The listing builds one solid part. Answer for the finished solid, in the listing's coordinates (mm). Face numbers are marked on the shaded views. Coordinates: 2 decimals unless noted, no trailing zeros. Order: outer loops, then holes, each group sorted by start corner. A loop starts at its lowest first (then second) coordinate and runs counter-clockwise, first axis right, second up. Notation, with made-up numbers: (73, 62.25) - (77, 62.25) arc R31 ccw to (77, 96.25) - close; hole circle Ø10 at (37.5, 76). An arc over 180 degrees is marked (long way). Use a Markdown table: item, result. Add a question column.
Item 1: Find the intervals of material crossed by line 1 along Y through (x, z) = (-76.2, 17.25); line 2 along Y through (x, z) = (68.5, 46); line 3 along X through (y, z) = (3, 30.5), in increasing order.
Item 2: The part is cut by section C-C, the plane y = -7. Give the vertices of the cut face in (x, z), then the cut area to 3 significant figures.
Item 3: Flat-ended cylindrical pins translate along their axes: P1, Ø12.5, axis at x = -75, y = -4, coming from the +Z side; P2, Ø1.9, axis at x = 76.2, y = 0, coming from the -Z side. Find the tip coordinate at first contact, or state that the pin passes through.
Item 4: The part is cut by section B-B, the plane x = -147.5. Give the vertices of the cut face in (y, z), then the cut area to 3 significant figures.
Item 5: The part is cut by section A-A, the plane z = 44.5. Give the vertices of the cut face in (x, y), then the cut area to 3 significant figures.
Item 6: The mould has two halves that part along Y. Classify the marked faces 1, 2, 3 and 4: released by +Y, released by -Y, zero draft, split by the parting line, or undercut.
from build123d import *

# Parameters (mm, degrees)
F0_W     = 381
F0_H     = 76.2
F1_DEPTH = 50.8
F2_W     = 330.2
F2_H     = 25.4
F3_DEPTH = 25.4
F5_D     = 3.175


with BuildPart() as f1:
    # F0 (on Top) → F1 (new body)
    with BuildSketch(Plane.XY):
        Rectangle(F0_W, F0_H)
    extrude(amount=F1_DEPTH)

    # F2 (on face) → F3 (cut)
    with BuildSketch(Plane.XY.offset(50.8)):
        Rectangle(F2_W, F2_H)
    extrude(amount=-F3_DEPTH, mode=Mode.SUBTRACT)

    # F5 (through all)
    with Locations(Plane(origin=(0, 0, 0), x_dir=(1, 0, 0), z_dir=(0, 0, -1))):
        with Locations((-76.2, 0), (76.2, 0)):
            Hole(F5_D / 2)


solid = f1.part
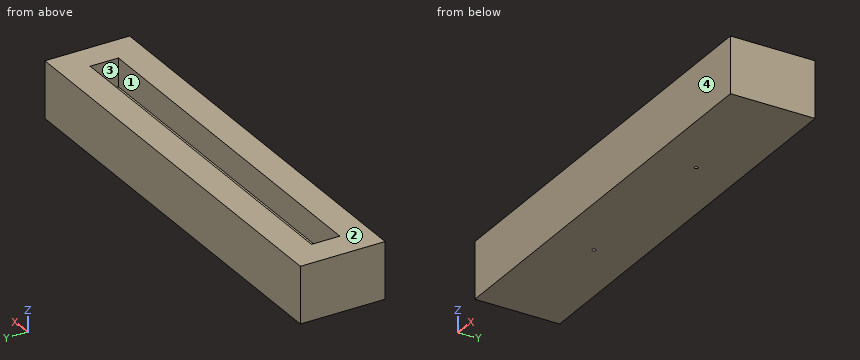
Solution:
| question | item | result |
|---|---|---|
| 1 | line 1 | y = -38.1 to -1.59, 1.59 to 38.1 |
| 1 | line 2 | y = -38.1 to -12.7, 12.7 to 38.1 |
| 1 | line 3 | x = -190.5 to -165.1, 165.1 to 190.5 |
| 2 | outline | (-190.5, 0) - (190.5, 0) - (190.5, 50.8) - (165.1, 50.8) - (165.1, 25.4) - (-165.1, 25.4) - (-165.1, 50.8) - (-190.5, 50.8) - close |
| 2 | area | 11,000 mm2 |
| 3 | P1 | stops at z = 25.4 |
| 3 | P2 | passes through |
| 4 | outline | (-38.1, 0) - (38.1, 0) - (38.1, 50.8) - (12.7, 50.8) - (12.7, 25.4) - (-12.7, 25.4) - (-12.7, 50.8) - (-38.1, 50.8) - close |
| 4 | area | 3,230 mm2 |
| 5 | outline | (-190.5, -38.1) - (190.5, -38.1) - (190.5, 38.1) - (-190.5, 38.1) - close; hole (-165.1, -12.7) - (165.1, -12.7) - (165.1, 12.7) - (-165.1, 12.7) - close |
| 5 | area | 20,600 mm2 |
| 6 | face 1 | undercut |
| 6 | face 2 | zero draft |
| 6 | face 3 | undercut |
| 6 | face 4 | released by -Y |
